Here's how the part is built. I have some questions about the finished solid (model axes, mm). Face numbers are marked on the shaded views. A direction names the side the tool comes from. Give positions to 0.01 mm unless a question says otherwise; leave off trailing zeros. Write each loop counter-clockwise with the first axis right and the second up, starting at its lowest first coordinate (ties: lowest second). Pieces come first, ordered by that corner, then holes. Notation, with made-up numbers: (45.25, 32.25) - (77.25, 32.25) arc R17 ccw to (77.25, 40.25) - close; hole circle Ø10 at (67, -16.5). An arc over 180 degrees is marked (long way). Use a Markdown table: item, result.
```python
from build123d import *

# Parameters (mm, degrees)
F0_R     = 2.15265
F0_R_2   = 11.1125
F1_DEPTH = 6.35
F2_R     = 14.2875
F2_R_2   = 11.1125
F3_DEPTH = 22.225
F5_DEPTH = 28.575
F6_R     = 1.7272
F7_DEPTH = 4.3100488316


# Not quite as in the source:
# - a fillet or chamfer that OpenCascade refuses, or shapes differently, is made with other operations: its cross-section is extruded or revolved along the edge and cut away or added


with BuildPart() as f1:
    # F0 (on Top) → F1 (new body)
    with BuildSketch(Plane.XY):
        with BuildLine():
            Line((6.6460049492, 12.6476588531), (4.6002217477, 20.2826257023))
            ThreePointArc((4.6002217477, 20.2826257023), (0, 23.8125), (-4.6002217477, 20.2826257023))
            Line((-4.6002217477, 20.2826257023), (-6.6460049492, 12.6476588531))
            ThreePointArc((-6.6460049492, 12.6476588531), (-10.1027881362, 10.1027881362), (-12.6476588531, 6.6460049492))
            Line((-12.6476588531, 6.6460049492), (-20.2826257023, 4.6002217477))
            ThreePointArc((-20.2826257023, 4.6002217477), (-23.8125, 0), (-20.2826257023, -4.6002217477))
            Line((-20.2826257023, -4.6002217477), (-12.6476588531, -6.6460049492))
            ThreePointArc((-12.6476588531, -6.6460049492), (-10.1027881362, -10.1027881362), (-6.6460049492, -12.6476588531))
            Line((-6.6460049492, -12.6476588531), (-4.6002217477, -20.2826257023))
            ThreePointArc((-4.6002217477, -20.2826257023), (0, -23.8125), (4.6002217477, -20.2826257023))
            Line((4.6002217477, -20.2826257023), (6.6460049492, -12.6476588531))
            ThreePointArc((6.6460049492, -12.6476588531), (10.1027881362, -10.1027881362), (12.6476588531, -6.6460049492))
            Line((12.6476588531, -6.6460049492), (20.2826257023, -4.6002217477))
            ThreePointArc((20.2826257023, -4.6002217477), (23.8125, 0), (20.2826257023, 4.6002217477))
            Line((20.2826257023, 4.6002217477), (12.6476588531, 6.6460049492))
            ThreePointArc((12.6476588531, 6.6460049492), (10.1027881362, 10.1027881362), (6.6460049492, 12.6476588531))
        make_face()
        with Locations((0, -19.05)):
            Circle(F0_R, mode=Mode.SUBTRACT)
        with Locations((-19.05, 0)):
            Circle(F0_R, mode=Mode.SUBTRACT)
        Circle(F0_R_2, mode=Mode.SUBTRACT)
        with Locations((19.05, 0)):
            Circle(F0_R, mode=Mode.SUBTRACT)
        with Locations((0, 19.05)):
            Circle(F0_R, mode=Mode.SUBTRACT)
    extrude(amount=F1_DEPTH)

    # F2 (on face) → F3 (join)
    with BuildSketch(Plane.XY.offset(6.35)):
        Circle(F2_R)
        Circle(F2_R_2, mode=Mode.SUBTRACT)
    extrude(amount=F3_DEPTH)

    # F4 (on face) → F5 (join, through all)
    with BuildSketch(Plane.XY.offset(28.575)):
        Polygon((-4.0671577888, -11.648290423), (-11.648290423, -4.0671577888), (-13.8933544533, -6.3122218191), (-6.3122218191, -13.8933544533), align=None)
    extrude(amount=-F5_DEPTH)

    # F6 (on face) → F7 (cut, up to face)
    with BuildSketch(Plane(origin=(-10.1027881362, -10.1027881362, 0), x_dir=(0.7071067812, -0.7071067812, 0), z_dir=(-0.7071067812, -0.7071067812, 0))):
        with Locations((0, 23.8125)):
            Circle(F6_R)
        with Locations((0, 4.7625)):
            Circle(F6_R)
    extrude(amount=-F7_DEPTH, mode=Mode.SUBTRACT)

    # F8: chamfer of 28.575 x 0.254 on 1 edges, made by hand

    # F8_s1 → F8_t2 (revolve, cut)
    with BuildSketch(Plane.XZ):
        Polygon((11.3665, 28.575), (11.1125, 0), (11.1125, 28.575), align=None)
    revolve(axis=Axis((0, 0, 28.575), (0, 0, -1)), mode=Mode.SUBTRACT)


solid = f1.part
```
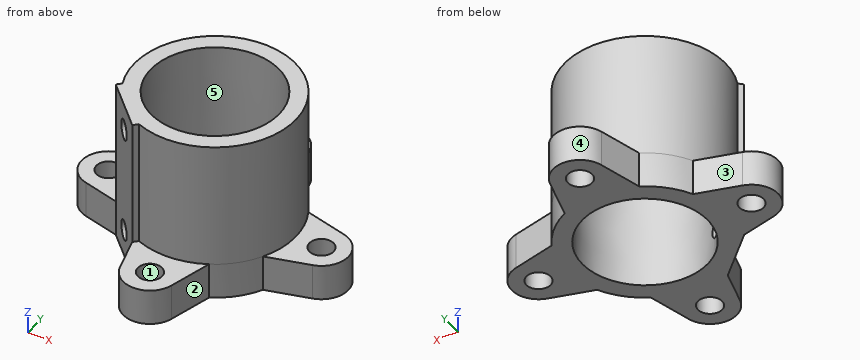
Item 1: Will these pins go through, and if not, where does the flat tip stop? pin 1 Ø1.5 at (x, z) = (12.5, 6.5) entering from +Y; pin 2 Ø3 at (y, z) = (2, 5) entering from +X; pin 3 Ø3.5 at (x, y) = (-16, 2.5) entering from +Z; pin 4 Ø12.5 at (x, y) = (17.5, 1) entering from +Z (3 decimals).
Values:
| item | result |
|---|---|
| pin 1 | stops at y = 8.13 |
| pin 2 | stops at x = 23.79 |
| pin 3 | stops at z = 6.35 |
| pin 4 | stops at z = 28.575 |
Item 2: For the marked faces 4 and 5, which set-ups out of +Z, -Z, +X, -X, +Y, -Y let a thin tool reach every point of the face, with its end or its side?
Values:
| item | result |
|---|---|
| face 4 | +Z, -Z, +Y |
| face 5 | +Z |
Item 3: Thinking about a two-plate mould opening in Y: for the marked faces 1, 2 and 3, which applies, +Y half, -Y half, draft (parallel to the pull), parting line (faces both ways), or undercut?
Values:
| item | result |
|---|---|
| face 1 | undercut |
| face 2 | -Y half |
| face 3 | +Y half |
Item 4: If we section it at D-D, the plane y = 16: Write out the boundary of the cut face in (x, z), plus the area to 3 significant figures.
Values:
| item | result |
|---|---|
| outline | (-5.75, 0) - (5.75, 0) - (5.75, 6.35) - (-5.75, 6.35) - close |
| area | 73.0 mm2 |
Item 5: If we section it at A-A, the plane y = -19.05: Write out the boundary of the cut face in (x, z), plus the area to 3 significant figures.
Values:
| item | result |
|---|---|
| outline | (-4.93, 0) - (-2.15, 0) - (-2.15, 6.35) - (-4.93, 6.35) - close; (2.15, 0) - (4.93, 0) - (4.93, 6.35) - (2.15, 6.35) - close |
| area | 35.3 mm2 |
Item 6: I need wall thicknesses on line 1 along Y through (x, z) = (-5, 10.75); line 2 along Y through (x, z) = (19.05, 1.5); line 3 along Z through (x, y) = (-2, 21.5). Which ranges of each line are inside material? Lowest first, please. Write a range as [from, to].
Values:
| item | result |
|---|---|
| line 1 | y = [-13.38, -10.03], [10.03, 13.38] |
| line 2 | y = [-4.93, -2.15], [2.15, 4.93] |
| line 3 | z = [0, 6.35] |
Item 7: If we section it at C-C, the plane z = 9.5: Write out the boundary of the cut face in (x, y) (1 decimal), plus the area to 3 significant figures.
Values:
| item | result |
|---|---|
| outline | (-13.9, -6.3) - (-6.3, -13.9) - (-5.6, -13.2) arc R14.3 ccw (long way) to (-13.2, -5.6) - close; hole circle Ø22.4 at (0, 0) |
| area | 251 mm2 |
